Input: dimensioned drawing with shaded views. Units: mm. Origin: part minimum x, y, z. Coordinates: 2 decimals unless noted, no trailing zeros. Loops run counter-clockwise (first coordinate to the right, second up) from the corner with the lowest first, then second, coordinate; pieces in that order, holes last.
Item 1: Line query: probe 1 along Y at (x, z) = (144, 2); probe 2 along X at (y, z) = (65, 0.45); probe 3 along Y at (x, z) = (93.5, 0.7). Output: solid intervals per line, ascending.
Item 2: Section query B-B, the plane z = 1.5. State how many separate pieces and enclosed holes the cut face has, then the cut area to 3 significant figures.
Item 3: Section query C-C, the plane y = 12. Return the cut outline in (x, z).
Item 4: Section query A-A, the plane y = 76.5. Return the cut outline in (x, z).
Item 5: Section query D-D, the plane x = 51.5. Return the cut outline in (y, z).
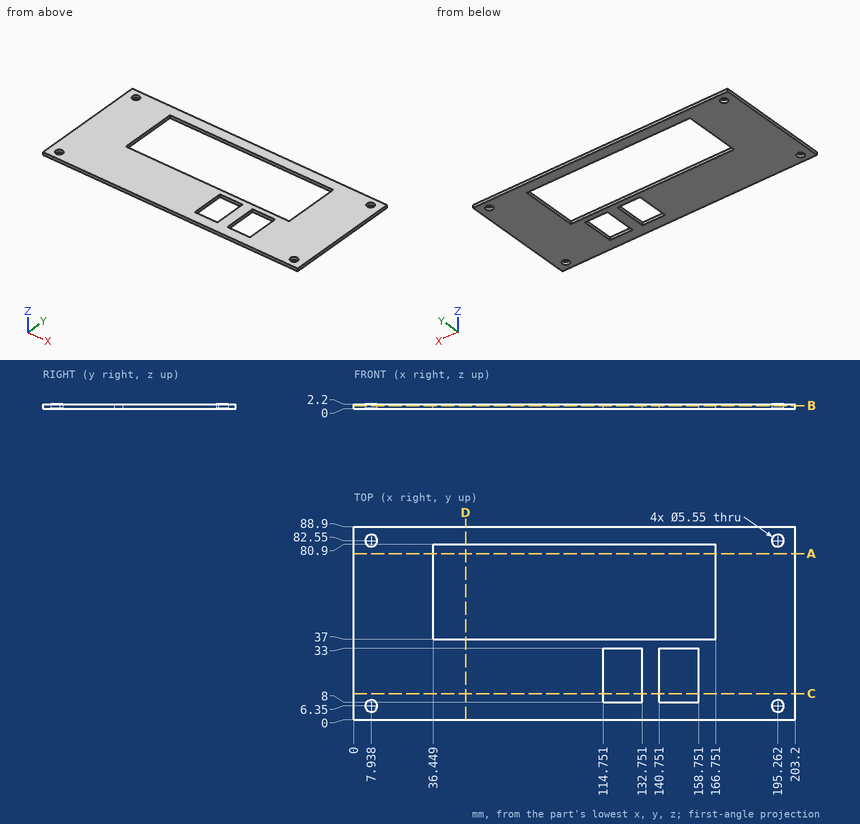
Verdict:
1. probe 1: y = 0 to 8, 33 to 37, 80.9 to 88.9
1. probe 2: x = 0 to 36.45, 166.75 to 203.2
1. probe 3: y = 0 to 37, 80.9 to 88.9
2. separate pieces: 1
2. enclosed holes: 7
2. area: 11,300 mm2
3. outline: (0, 0) - (114.75, 0) - (114.75, 2.2) - (0, 2.2) - close; (132.75, 0) - (140.75, 0) - (140.75, 2.2) - (132.75, 2.2) - close; (158.75, 0) - (203.2, 0) - (203.2, 2.2) - (158.75, 2.2) - close
4. outline: (0, 0) - (36.45, 0) - (36.45, 2.2) - (0, 2.2) - close; (166.75, 0) - (203.2, 0) - (203.2, 2.2) - (166.75, 2.2) - close
5. outline: (0, 0) - (37, 0) - (37, 2.2) - (0, 2.2) - close; (80.9, 0) - (88.9, 0) - (88.9, 2.2) - (80.9, 2.2) - close
